Here's the drawing with two shaded views (mm, measured from the low corner). I have some questions. A direction names the side the tool comes from. Coordinates: 2 decimals unless noted, no trailing zeros. Write each loop counter-clockwise with the first axis right and the second up, starting at its lowest first coordinate (ties: lowest second). Pieces come first, ordered by that corner, then holes. Notation, with made-up numbers: (-17.75, 26.5) -> (-10.75, 26.5) arc R28 ccw to (-10.75, 47.5) -> close; hole circle Ø7 at (-24.75, 41.25). An arc over 180 degrees is marked (long way). Use one line per item in the form item = value.
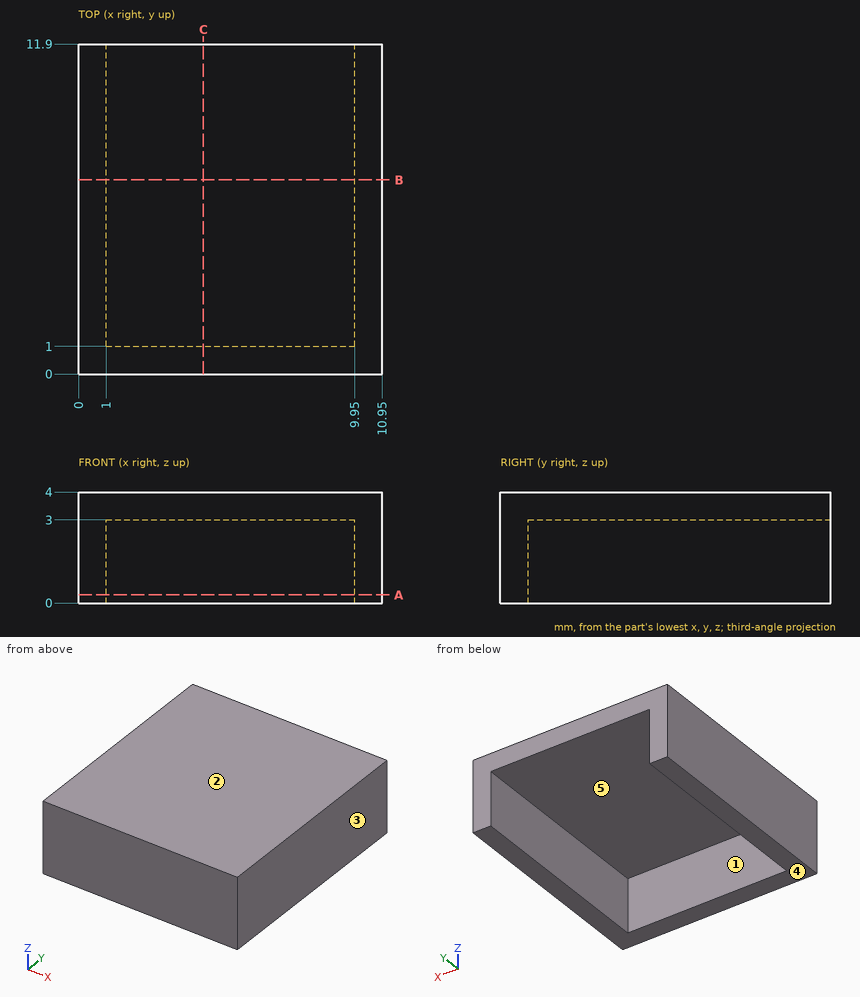
Q1. For the marked faces 4 and 5, which set-ups out of +Z, -Z, +X, -X, +Y, -Y let a thin tool reach every point of the face, with its end or its side?
Return value:
face_4 = -Z, +X, -X, +Y, -Y
face_5 = -Z, +Y
Q2. Suppose I cut it at C-C (x = 4.5). Write out the boundary of the cut face in (y, z), then the cut area to 3 significant figures.
Return value:
outline = (0, 0) -> (1, 0) -> (1, 3) -> (11.9, 3) -> (11.9, 4) -> (0, 4) -> close
area = 14.9 mm2
Q3. Thinking about a two-plate mould opening in X: for the marked faces 1, 2 and 3, which applies, released by +X, released by -X, zero draft, split by the parting line, or undercut?
Return value:
face_1 = undercut
face_2 = zero draft
face_3 = released by +X
Q4. Suppose I cut it at B-B (y = 7). Write out the boundary of the cut face in (x, z).
Return value:
outline = (0, 0) -> (1, 0) -> (1, 3) -> (9.95, 3) -> (9.95, 0) -> (10.95, 0) -> (10.95, 4) -> (0, 4) -> close
Q5. Will these pins go through, and if not, where does the flat tip stop? pin 1 (4.5 mm diameter, centred on x = 7.5, y = 7.5, fed in from -Z); pin 2 (0.9 mm diameter, centred on x = 7, z = 1.5, fed in from +Y).
Return value:
pin_1 = 3
pin_2 = 1
Q6. Suppose I cut it at A-A (z = 0.3). Write out the boundary of the cut face in (x, y), then the cut area to 4 significant figures.
Return value:
outline = (0, 0) -> (10.95, 0) -> (10.95, 11.9) -> (9.95, 11.9) -> (9.95, 1) -> (1, 1) -> (1, 11.9) -> (0, 11.9) -> close
area = 32.75 mm2
Q7. If I drill on line 1 (X direction, y = 4.25, z = 1.3); line 2 (Z direction, x = 4, y = 4.5); line 3 (Y direction, x = 4.75, z = 2.5), over which ranges is the centre line in solid material (lowest first)? Write a range as from..to.
Return value:
line_1 = 0..1, 9.95..10.95
line_2 = 3..4
line_3 = 0..1
